```python
from build123d import *

# Parameters (mm, degrees)
SKETCH1_W           = 40
SKETCH1_H           = 20
BOSS_EXTRUDE1_DEPTH = 1.5
SKETCH2_R           = 1.5
BOSS_EXTRUDE3_DEPTH = 1.5
SKETCH3_R           = 1
CUT_EXTRUDE1_DEPTH  = 1.5
SKETCH4_W           = 5.5
SKETCH4_H           = 10
BOSS_EXTRUDE4_DEPTH = 7
SKETCH5_W           = 26
SKETCH5_H           = 15
BOSS_EXTRUDE5_DEPTH = 7


with BuildPart() as part:
    # Sketch1 → Boss-Extrude1 (new body)
    with BuildSketch(Plane(origin=(0, 0, 0), x_dir=(1, 0, 0), z_dir=(0, 1, 0))):
        Rectangle(SKETCH1_W, SKETCH1_H)
    extrude(amount=BOSS_EXTRUDE1_DEPTH)

    # Sketch2 → Boss-Extrude3 (add)
    with BuildSketch(Plane(origin=(0, 1.5, 0), x_dir=(1, 0, 0), z_dir=(0, 1, 0))):
        with Locations((-10, 10)):
            Circle(SKETCH2_R)
        with Locations((-10, -10)):
            Circle(SKETCH2_R)
        with Locations((20, 0)):
            Circle(SKETCH2_R)
    extrude(amount=-BOSS_EXTRUDE3_DEPTH)

    # Sketch3 → Cut-Extrude1 (cut)
    with BuildSketch(Plane(origin=(0, 1.5, 0), x_dir=(1, 0, 0), z_dir=(0, 1, 0))):
        with Locations((-10, -10)):
            Circle(SKETCH3_R)
        with Locations((20, 0)):
            Circle(SKETCH3_R)
        with Locations((-10, 10)):
            Circle(SKETCH3_R)
    extrude(amount=-CUT_EXTRUDE1_DEPTH, mode=Mode.SUBTRACT)

    # Sketch4 → Boss-Extrude4 (add)
    with BuildSketch(Plane(origin=(0, 1.5, 0), x_dir=(1, 0, 0), z_dir=(0, 1, 0))):
        with Locations((-16.25, 0)):
            Rectangle(SKETCH4_W, SKETCH4_H)
    extrude(amount=BOSS_EXTRUDE4_DEPTH)

    # Sketch5 → Boss-Extrude5 (add)
    with BuildSketch(Plane(origin=(0, 1.5, 0), x_dir=(1, 0, 0), z_dir=(0, 1, 0))):
        with Locations((5, 0.53388581)):
            Rectangle(SKETCH5_W, SKETCH5_H)
    extrude(amount=BOSS_EXTRUDE5_DEPTH)


solid = part.part
```
Can you work these out from the model? Positions are in its coordinate system, mm. A direction names the side the tool comes from. Coordinates: 2 decimals unless noted, no trailing zeros. Loops run counter-clockwise (first coordinate to the right, second up) from the corner with the lowest first, then second, coordinate; pieces in that order, holes last. Notation, with made-up numbers: (25.25, 19) -> (39.25, 19) arc R16 ccw to (39.25, 45) -> close; hole circle Ø2 at (77, 69). An arc over 180 degrees is marked (long way). Put each result on its own line as item: value. Start each with the question number.
Q1. Thinking about a two-plate mould opening in Z: for faces 1 (the face through (-10, 1, 9)), 2 (the face through (-16, 1, 10)), 3 (the face through (-13.5, 5, 0)), 4 (the face through (5, 5, -8.034)), which applies, pulls with the +Z half, pulls with the -Z half, needs draft (parallel to the pull), parting line crosses it, or undercut?
Q2. I want a section at B-B (z = 0). Write out the boundary of the cut face in (x, y).
Q3. I want a section at D-D (x = -15). Write out the boundary of the cut face in (y, z).
Q4. If I drill on line 1 (X direction, y = 0.75, z = 0); line 2 (X direction, y = 3.5, z = -1.5); line 3 (Y direction, x = 2.5, z = 8.25), over which ranges is the centre line in solid material (lowest first)? Write a range as [from, to].
Q5. I'm going to push flat-ended pins straight in: P1, Ø2, axis at y = 4.5, z = 1.5, coming from the +X side; P2, Ø1, axis at x = -16, y = 3, coming from the -Z side; P3, Ø2, axis at y = 1, z = -4, coming from the +X side. Where does each tip first touch, or does it pass through?
Q6. For faces 5 (the face through (20, 1, -6)), 6 (the face through (-16, 5, -5)), 7 (the face through (6, 1, 10)), which set-ups out of +Z, -Z, +X, -X, +Y, -Y let a thin tool reach every point of the face, with its end or its side?
Q7. I want a section at C-C (y = 6). Write out the boundary of the cut face in (x, z).
Q8. I want a section at A-A (x = -10). Write out the boundary of the cut face in (y, z).
Taken from the geometry:
1. face 1: undercut
1. face 2: pulls with the +Z half
1. face 3: needs draft
1. face 4: pulls with the -Z half
2. outline: (-20, 0) -> (19, 0) -> (19, 1.5) -> (18, 1.5) -> (18, 8.5) -> (-8, 8.5) -> (-8, 1.5) -> (-13.5, 1.5) -> (-13.5, 8.5) -> (-19, 8.5) -> (-19, 1.5) -> (-20, 1.5) -> close; (21, 0) -> (21.5, 0) -> (21.5, 1.5) -> (21, 1.5) -> close
3. outline: (0, -10) -> (1.5, -10) -> (1.5, -5) -> (8.5, -5) -> (8.5, 5) -> (1.5, 5) -> (1.5, 10) -> (0, 10) -> close
4. line 1: x = [-20, 19], [21, 21.5]
4. line 2: x = [-19, -13.5], [-8, 18]
4. line 3: y = [0, 1.5]
5. P1: stops at x = 18
5. P2: stops at z = -5
5. P3: stops at x = 20
6. face 5: -Z, +X, +Y, -Y
6. face 6: -Z, -X, +Y
6. face 7: +Z, +X, +Y, -Y
7. outline: (-19, -5) -> (-13.5, -5) -> (-13.5, 5) -> (-19, 5) -> close; (-8, -8.03) -> (18, -8.03) -> (18, 6.97) -> (-8, 6.97) -> close
8. outline: (0, -11.5) -> (1.5, -11.5) -> (1.5, -11) -> (0, -11) -> close; (0, -9) -> (1.5, -9) -> (1.5, 9) -> (0, 9) -> close; (0, 11) -> (1.5, 11) -> (1.5, 11.5) -> (0, 11.5) -> close
